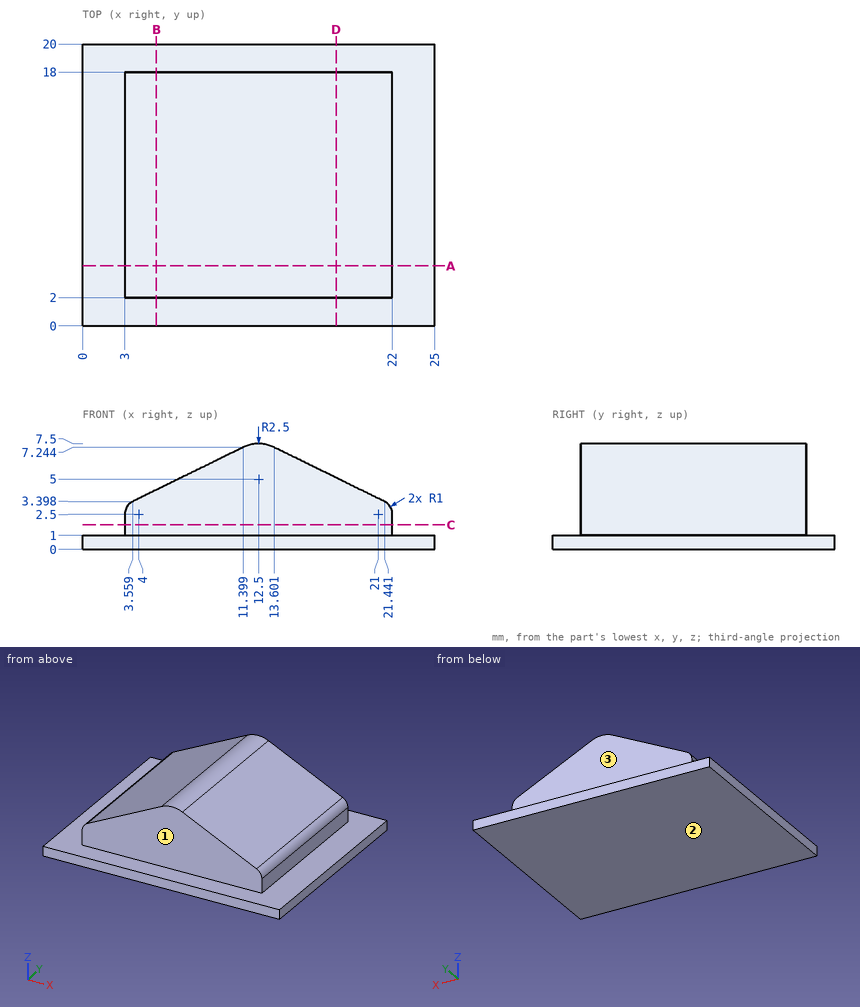
For this review, use the dimensioned drawing (mm, ordinates from the lowest corner) and the shaded views. A direction names the side the tool comes from. Round coordinates to 2 decimals unless told otherwise and drop trailing zeros. Order: outer loops, then holes, each group sorted by start corner. A loop starts at its lowest first (then second) coordinate and runs counter-clockwise, first axis right, second up. Notation, with made-up numbers: M 73,-20.75 L 108,-20.75 A16 cw 108,-4.75 Z; hole C 51,74.5 d7. An arc over 180 degrees is marked long. Write each question's results on one line, items separated by ' | '. Start each with the question number.
1. Add section B-B (x = 5.25). State the section outline as (y, z) points.
2. Add section D-D (x = 18). State the section outline as (y, z) points (1 decimal).
3. Tool access review of the marked faces 1, 2 and 3: name each direction out of +Z, -Z, +X, -X, +Y, -Y from which nothing blocks a thin tool from reaching the whole face with its end or side.
4. To check wall thickness, follow L1, parallel to Y at x = 18.5, z = 2; L2, parallel to X at y = 16, z = 2.5; L3, parallel to X at y = 13, z = 5.5 (1 decimal). State the ranges of each line that lie inside material, in increasing order. Write a range as [from, to].
5. Add section A-A (y = 4.25). State the section outline as (x, z) points (1 decimal).
6. Add section C-C (z = 1.75). State the section outline as (x, y) points, then the cut area to 3 significant figures.
7. Clearance check with flat-ended pins moving along their axes: pin 1 Ø6 at (x, y) = (17, 13.5) entering from +Z; pin 2 Ø0.8 at (y, z) = (9, 2) entering from +X; pin 3 Ø1.5 at (x, z) = (3.5, 3) entering from -Y. State where each tip first meets the part, or that it passes through.
Output values:
1) outline: M 0,0 L 20,0 L 20,1 L 18,1 L 18,4.23 L 2,4.23 L 2,1 L 0,1 Z
2) outline: M 0,0 L 20,0 L 20,1 L 18,1 L 18,5.1 L 2,5.1 L 2,1 L 0,1 Z
3) face 1: +Z, +X, -X, -Y | face 2: -Z, +X, -X, +Y, -Y | face 3: +Z, +X, -X, +Y
4) L1: [2, 18] | L2: [3, 22] | L3: [7.8, 17.2]
5) outline: M 0,0 L 25,0 L 25,1 L 22,1 L 22,2.5 A1 ccw 21.4,3.4 L 13.6,7.2 A2.5 ccw 11.4,7.2 L 3.6,3.4 A1 ccw 3,2.5 L 3,1 L 0,1 Z
6) outline: M 3,2 L 22,2 L 22,18 L 3,18 Z | area: 304 mm^2
7) pin 1: z = 7.05 | pin 2: x = 22 | pin 3: y = 2
